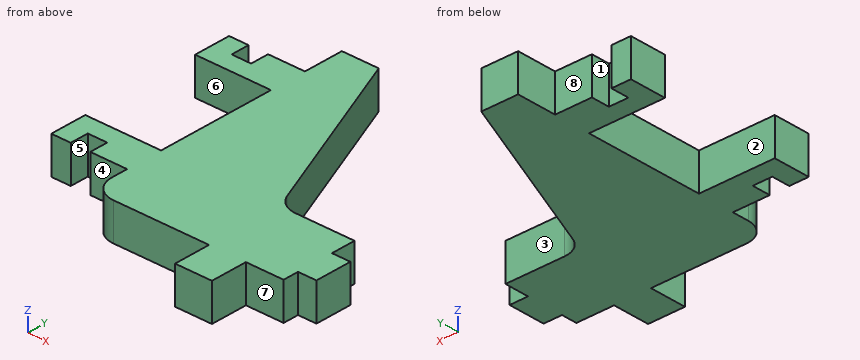
```python
from build123d import *

# Parameters (mm, degrees)
BOSS_EXTRUDE1_DEPTH = 6
FILLET1_R           = 3.81


with BuildPart() as part:
    # Sketch1 → Boss-Extrude1 (new body)
    with BuildSketch(Plane.XY):
        Polygon((-12.35, 31.925), (0, 31.925), (0, 37.925), (-6, 37.925), (-6, 34.925), (-9.175, 34.925), (-9.175, 37.925), (-12.35, 37.925), align=None)
        Polygon((19.3548, 12.525), (31.496, 12.525), (31.496, 8.54), (34.496, 8.54), (34.496, 2.54), (31.496, 2.54), (31.496, 0), (25.3548, 0), (25.3548, -6), (19.3548, -6), (19.3548, 0), (0, 0), (0, 44.45), (6, 44.45), align=None)
        Polygon((-6, 6.525), (0, 6.525), (0, 12.525), (-12.35, 12.525), (-12.35, 6.525), (-9.175, 6.525), (-9.175, 9.525), (-6, 9.525), align=None)
    extrude(amount=BOSS_EXTRUDE1_DEPTH)

    # Fillet1
    fillet1_edges = [part.edges().sort_by_distance(p)[0] for p in [
        (19.3548, 12.525, 3),
        (0, 0, 3),
    ]]
    fillet(fillet1_edges, radius=FILLET1_R)


solid = part.part
```
Can you work these out from the model? Positions are in its coordinate system, mm. Face numbers are marked on the shaded views. A direction names the side the tool comes from. Coordinates: 2 decimals unless noted, no trailing zeros. Loops run counter-clockwise (first coordinate to the right, second up) from the corner with the lowest first, then second, coordinate; pieces in that order, holes last. Notation, with made-up numbers: (36.5, 23) - (83.5, 23) arc R14 ccw to (83.5, 28) - close; hole circle Ø6 at (21.25, 72). An arc over 180 degrees is marked (long way). Answer as CSV lines item,"result". Start each with the question number.
1) I need wall thicknesses on line 1 (Y direction, x = 23, z = 2.2) (3 decimals); line 2 (X direction, y = 11.5, z = 1.45); line 3 (Y direction, x = 5.5, z = 5.8). Which ranges of each line are inside material? Lowest first, please. Write a range as from..to.
2) Which directions (+Z, -Z, +X, -X, +Y, -Y) give clear straight access to the entire face, cutting with the end or side of a thin tool? Please do the marked faces 4, 5, 6, 7 and 8.
3) Suppose I cut it at C-C (y = 35.5). Please give me the cut outline in (x, z) (3 decimals), plus the area to 3 significant figures.
4) For pin 1 (2.5 mm diameter, centred on x = 32.5, z = 3, fed in from -Y); pin 2 (5 mm diameter, centred on x = -5.5, y = 36.5, fed in from -Z); pin 3 (0.8 mm diameter, centred on y = 1, z = 2, fed in from +X); pin 4 (3 mm diameter, centred on x = -4.5, z = 4.5, fed in from +Y) (3 decimals), each with a flat end and sliding along its axis, tell me the tip position at first contact or that it passes through.
5) Thinking about a two-plate mould opening in Y: for the marked faces 1, 2 and 3, which applies, pulls with the +Y half, pulls with the -Y half, needs draft (parallel to the pull), parting line crosses it, or undercut?
6) Suppose I cut it at A-A (x = -8). Please give me the cut outline in (y, z) (3 decimals), plus the area to 3 significant figures.
7) Suppose I cut it at D-D (x = 24.5). Please give me the cut outline in (y, z) (3 decimals).
Check result:
1,line 1,"y = -6..12.525"
1,line 2,"x = -12.35..31.5"
1,line 3,"y = 0..44.45"
2,face 4,"+Z, -Z, -X, -Y"
2,face 5,"+Z, -Z, -Y"
2,face 6,"+Z, -Z, -X"
2,face 7,"+Z, -Z, +X, -Y"
2,face 8,"+Z, -Z, -X, +Y"
3,outline,"(-12.35, 0) - (-9.175, 0) - (-9.175, 6) - (-12.35, 6) - close; (-6, 0) - (9.744, 0) - (9.744, 6) - (-6, 6) - close"
3,area,"114 mm²"
4,pin 1,"stops at y = 0"
4,pin 2,"stops at z = 0"
4,pin 3,"stops at x = 31.5"
4,pin 4,"stops at y = 37.925"
5,face 1,"needs draft"
5,face 2,"undercut"
5,face 3,"pulls with the +Y half"
6,outline,"(9.525, 0) - (12.525, 0) - (12.525, 6) - (9.525, 6) - close; (31.925, 0) - (34.925, 0) - (34.925, 6) - (31.925, 6) - close"
6,area,"36.0 mm²"
7,outline,"(-6, 0) - (12.525, 0) - (12.525, 6) - (-6, 6) - close"
